Build history of the part. All positions in model axes, mm. A direction names the side the tool comes from. Give positions to 0.01 mm unless a question says otherwise; leave off trailing zeros. Write each loop counter-clockwise with the first axis right and the second up, starting at its lowest first coordinate (ties: lowest second). Pieces come first, ordered by that corner, then holes. Notation, with made-up numbers: (82, 73) -> (135, 73) arc R11 ccw to (135, 91) -> close; hole circle Ø2 at (-36, 57.5). An arc over 180 degrees is marked (long way). Put each result on its own line as item: value. Start each with the question number.
Item 1: Slice it at D-D, the plane x = -19.5. List the corners of the cut face in (y, z).
Item 2: Slice it at A-A, the plane y = -17. List the corners of the cut face in (x, z).
Item 3: Drill centre lines: line 1 along X through (y, z) = (-5, 1.65); line 2 along Y through (x, z) = (-11, 0.55); line 3 along X through (y, z) = (55, 4.15). Where is each one in solid material? Low to high.
Item 4: Flat gauge pins, fed straight in: pin 1 Ø1.7 at (x, z) = (8, 3.5) entering from +Y; pin 2 Ø1.7 at (x, z) = (11.5, 3.5) entering from -Y; pin 3 Ø1.4 at (x, y) = (-43.84, 36.6) entering from +Z. Where does each tip first touch, or does it go through?
Item 5: Slice it at C-C, the plane z = 2.85. Give the number of separate pieces and of enclosed holes in the cut face, plus the area to 3 significant figures.
Item 6: Slice it at B-B, the plane x = 1.5. List the corners of the cut face in (y, z), plus the area to 3 significant figures.
Item 7: Tool access for faces 5 (the flat face through (0, -60.401, 3)), 6 (the flat face through (12, -20.134, 3)), 7 (the flat face through (4.936, 57, 3)): list every direction of +Z, -Z, +X, -X, +Y, -Y with a clear straight run to the whole face (end or side of a thin tool).
Item 8: Two-plate mould, pull along X, no slides. Class faces 1 (the flat face through (-14.808, -58, 3)), 2 (the flat face through (-14, 60.401, 3)), 3 (the flat face through (-27.508, -68, 3)), 4 (the flat face through (-14.808, 0, 3)): pulls with the +X half, pulls with the -X half, needs draft (parallel to the pull), parting line crosses it, or undercut.
```python
from build123d import *

# Parameters (mm, degrees)
SKETCH1_W           = 29.6164
SKETCH1_H           = 120.8024
BOSS_EXTRUDE1_DEPTH = 5.7912
SKETCH3_W           = 5.7912
SKETCH3_H           = 40.267466666
CUT_EXTRUDE2_DEPTH  = 63.458992516
SKETCH6_W           = 9.872133334
SKETCH6_H           = 5.7912
CUT_EXTRUDE5_DEPTH  = 63.458992516
SKETCH9_W           = 5.7912
SKETCH9_H           = 120.8024
BOSS_EXTRUDE3_DEPTH = 44.45
SKETCH13_W          = 31.75
SKETCH13_H          = 5.7912
BOSS_EXTRUDE4_DEPTH = 25.4
SKETCH14_W          = 31.75
SKETCH14_H          = 5.7912
BOSS_EXTRUDE5_DEPTH = 25.4
SKETCH16_R          = 2.4003
SKETCH16_R_2        = 1.905
CUT_EXTRUDE8_DEPTH  = 13.462
SKETCH18_R          = 1.1938
CUT_EXTRUDE9_DEPTH  = 105.436191936
FILLET2_R           = 15.24
FILLET3_R           = 5.08
CAVITY1_START       = -14.8082
CAVITY1_OUTLINE_W   = 5.7912
CAVITY1_OUTLINE_H   = 5.7912
CAVITY1_DEPTH       = 9.872133333
CAVITY1_START_2     = 4.936066667
CAVITY1_2_OUTLINE_W = 5.7912
CAVITY1_2_OUTLINE_H = 5.7912
CAVITY1_2_DEPTH     = 9.872133333


# Read off the part's stored shape, not the designer's step: Cavity1
with BuildPart() as part:
    # Sketch1 → Boss-Extrude1 (new body)
    with BuildSketch(Plane.XY):
        Rectangle(SKETCH1_W, SKETCH1_H)
    extrude(amount=BOSS_EXTRUDE1_DEPTH)

    # Sketch3 → Cut-Extrude2 (cut, through all)
    with BuildSketch(Plane(origin=(0, 0, 0), x_dir=(-1, 0, 0), z_dir=(0, 0, -1))):
        with Locations((-11.9126, 0)):
            Rectangle(SKETCH3_W, SKETCH3_H)
        with Locations((11.9126, 0)):
            Rectangle(SKETCH3_W, SKETCH3_H)
    extrude(amount=-CUT_EXTRUDE2_DEPTH, mode=Mode.SUBTRACT)

    # Sketch6 → Cut-Extrude5 (cut, through all)
    with BuildSketch(Plane(origin=(0, 0, 0), x_dir=(-1, 0, 0), z_dir=(0, 0, -1))):
        with Locations((0, 57.5056)):
            Rectangle(SKETCH6_W, SKETCH6_H)
    extrude(amount=-CUT_EXTRUDE5_DEPTH, mode=Mode.SUBTRACT)

    # Sketch9 → Boss-Extrude3 (add)
    with BuildSketch(Plane.ZY.offset(14.8082)):
        with Locations((2.8956, 0)):
            Rectangle(SKETCH9_W, SKETCH9_H)
    extrude(amount=BOSS_EXTRUDE3_DEPTH)

    # Sketch13 → Boss-Extrude4 (add)
    with BuildSketch(Plane.XZ.offset(60.4012)):
        with Locations((-43.3832, 2.8956)):
            Rectangle(SKETCH13_W, SKETCH13_H)
    extrude(amount=BOSS_EXTRUDE4_DEPTH)

    # Sketch14 → Boss-Extrude5 (add)
    with BuildSketch(Plane(origin=(0, 60.4012, 0), x_dir=(1, 0, 0), z_dir=(0, 1, 0))):
        with Locations((-43.3832, -2.8956)):
            Rectangle(SKETCH14_W, SKETCH14_H)
    extrude(amount=BOSS_EXTRUDE5_DEPTH)

    # Sketch16 → Cut-Extrude8 (cut)
    with BuildSketch(Plane.XY):
        with Locations(Location((-43.842108599, -6.4897, 0), (0, 0, 180))):
            Circle(SKETCH16_R)
        with Locations(Location((-43.842108599, 6.985, 0), (0, 0, 180))):
            Circle(SKETCH16_R_2)
    extrude(amount=CUT_EXTRUDE8_DEPTH, mode=Mode.SUBTRACT)

    # Sketch18 → Cut-Extrude9 (cut, through all)
    with BuildSketch(Plane(origin=(0, 0, 0), x_dir=(-1, 0, 0), z_dir=(0, 0, -1))):
        with Locations((43.842108599, 48.8696)):
            Circle(SKETCH18_R)
        with Locations((43.842108599, 36.6014)):
            Circle(SKETCH18_R)
        with Locations((43.842108599, -49.5808)):
            Circle(SKETCH18_R)
        with Locations((43.842108599, -61.849)):
            Circle(SKETCH18_R)
    extrude(amount=-CUT_EXTRUDE9_DEPTH, mode=Mode.SUBTRACT)

    # Fillet2
    fillet2_edges = [part.edges().sort_by_distance(p)[0] for p in [
        (-27.5082, 85.8012, 2.8956),
        (-27.5082, -85.8012, 2.8956),
        (-59.2582, 85.8012, 2.8956),
        (-59.2582, -85.8012, 2.8956),
    ]]
    fillet(fillet2_edges, radius=FILLET2_R)

    # Fillet3
    fillet3_edges = [part.edges().sort_by_distance(p)[0] for p in [
        (-27.5082, -60.4012, 2.8956),
        (-27.5082, 60.4012, 2.8956),
    ]]
    fillet(fillet3_edges, radius=FILLET3_R)

    # Cavity1 outline → Cavity1 (cut)
    with BuildSketch(Plane.YZ.offset(CAVITY1_START)):
        with Locations((-57.5056, 2.8956)):
            Rectangle(CAVITY1_OUTLINE_W, CAVITY1_OUTLINE_H)
    extrude(amount=CAVITY1_DEPTH, mode=Mode.SUBTRACT)

    # Cavity1 2 outline → Cavity1 2 (cut)
    with BuildSketch(Plane.YZ.offset(CAVITY1_START_2)):
        with Locations((-57.5056, 2.8956)):
            Rectangle(CAVITY1_2_OUTLINE_W, CAVITY1_2_OUTLINE_H)
    extrude(amount=CAVITY1_2_DEPTH, mode=Mode.SUBTRACT)


solid = part.part
```
Values follow:
1. outline: (-60.4, 0) -> (60.4, 0) -> (60.4, 5.79) -> (-60.4, 5.79) -> close
2. outline: (-59.26, 0) -> (-14.81, 0) -> (-14.81, 5.79) -> (-59.26, 5.79) -> close; (-9.02, 0) -> (9.02, 0) -> (9.02, 5.79) -> (-9.02, 5.79) -> close
3. line 1: -59.26 to -45.72, -41.96 to -14.81, -9.02 to 9.02
3. line 2: -54.61 to -20.13, 20.13 to 60.4
3. line 3: -59.26 to -4.94, 4.94 to 14.81
4. pin 1: y = 60.4
4. pin 2: y = -54.61
4. pin 3: through
5. separate pieces: 1
5. enclosed holes: 7
5. area: 9,690 mm2
6. outline: (-60.4, 0) -> (54.61, 0) -> (54.61, 5.79) -> (-60.4, 5.79) -> close
6. area: 666 mm2
7. face 5: +Z, -Z, +X, -Y
7. face 6: +Z, -Z, +X
7. face 7: +Z, -Z, +Y
8. face 1: undercut
8. face 2: needs draft
8. face 3: pulls with the +X half
8. face 4: undercut
